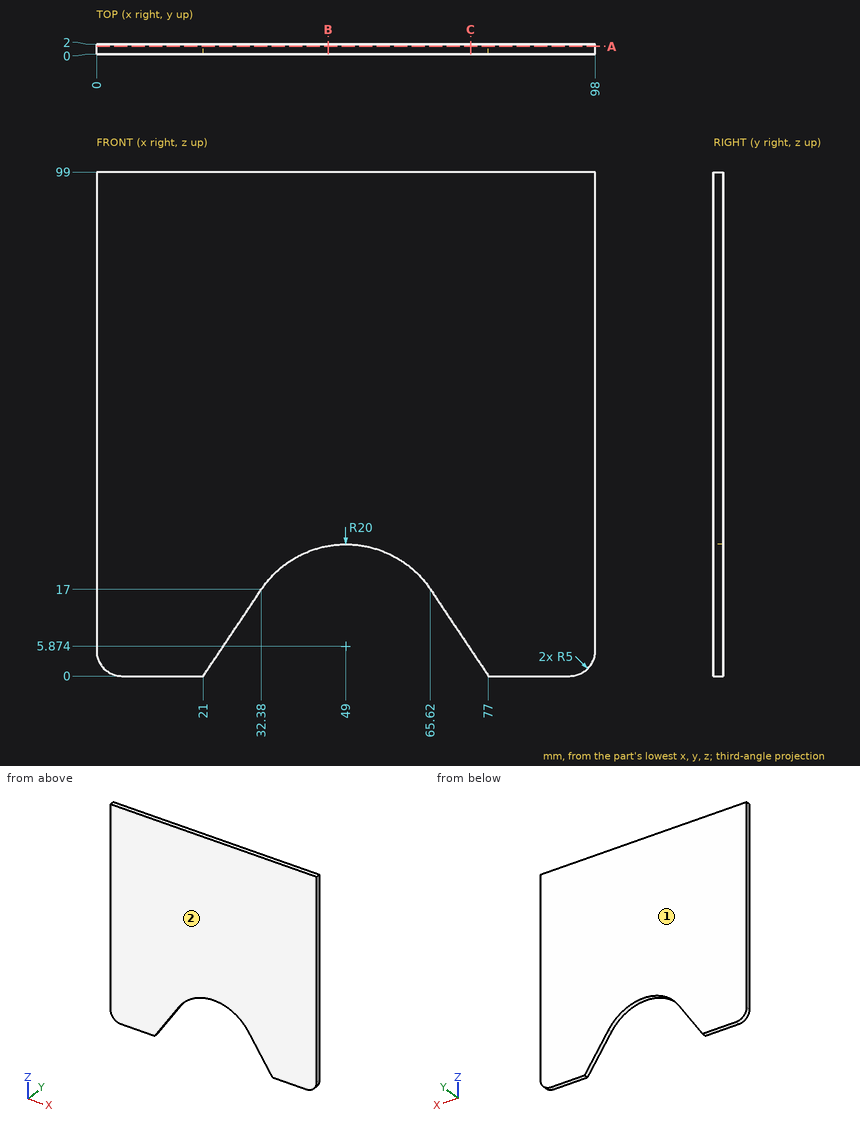
Source: three-view drawing plus pictorial views. Frame: mm from the lowest corner of the part. Coordinates: 2 decimals unless noted, no trailing zeros. Order: outer loops, then holes, each group sorted by start corner. A loop starts at its lowest first (then second) coordinate and runs counter-clockwise, first axis right, second up. Notation, with made-up numbers: M -10,14 L 19,14 A20 ccw 19,38 Z; hole C 70.25,30 d3. An arc over 180 degrees is marked long. Answer in a Markdown table with one row per item.
(1) Section query B-B, the plane x = 45.5. Output: boundary loops of the cut face in (y, z), plus the area to 3 significant figures.
Numbers:
| item | result |
|---|---|
| outline | M 0,25.57 L 2,25.57 L 2,99 L 0,99 Z |
| area | 147 mm^2 |
(2) Section query C-C, the plane x = 73.5. Output: boundary loops of the cut face in (y, z).
Numbers:
| item | result |
|---|---|
| outline | M 0,5.23 L 2,5.23 L 2,99 L 0,99 Z |
(3) Section query A-A, the plane y = 1.55. Output: boundary loops of the cut face in (x, z) (1 decimal).
Numbers:
| item | result |
|---|---|
| outline | M 0,5 A5 ccw 5,0 L 21,0 L 32.4,17 A20 cw 65.6,17 L 77,0 L 93,0 A5 ccw 98,5 L 98,99 L 0,99 Z |
(4) Material intervals for line 1 (X direction, y = 0.7, z = 10.5); line 2 (X direction, y = 0.2, z = 14); line 3 (Z direction, x = 73, y = 1.05) (1 decimal), sorted ascending. Write a range as [from, to].
Numbers:
| item | result |
|---|---|
| line 1 | x = [0, 28.03], [69.97, 98] |
| line 2 | x = [0, 30.37], [67.63, 98] |
| line 3 | z = [6, 99] |
(5) Draft query along Y for the marked faces 1 and 2. Return one class per face: pulls with the +Y half, pulls with the -Y half, needs draft (parallel to the pull), parting line crosses it, or undercut.
Numbers:
| item | result |
|---|---|
| face 1 | pulls with the +Y half |
| face 2 | pulls with the -Y half |
